Part model, mm, in its own coordinate system. A direction names the side the tool comes from. Coordinates: 2 decimals unless noted, no trailing zeros. Write each loop counter-clockwise with the first axis right and the second up, starting at its lowest first coordinate (ties: lowest second). Pieces come first, ordered by that corner, then holes. Notation, with made-up numbers: (16, -24.75) - (71, -24.75) arc R13 cw to (71, -16.75) - close; hole circle Ø1 at (-14, 43). An arc over 180 degrees is marked (long way). Write each question's results on one line, items separated by ' | '.
Autodesk Inventor part; units mm, degrees
ref_plane "YZ Plane" through (0, 0, 0) normal (1, 0, 0) x (0, 1, 0)
ref_plane "XZ Plane" through (0, 0, 0) normal (0, 1, 0) x (-1, 0, 0)
ref_plane "XY Plane" through (0, 0, 0) normal (0, 0, 1) x (1, 0, 0)
sketch "Sketch1" plane through (0, 0, 0) normal (0, 1, 0) x (-1, 0, 0)
  line L0 (-10.2591, 9.049) -> (9.7409, 9.049)
  line L1 (9.7409, 9.049) -> (9.7409, -10.951)
  line L2 (9.7409, -10.951) -> (-10.2591, -10.951)
  line L3 (-10.2591, -10.951) -> (-10.2591, 9.049)
  point P0 (0, 0)
  dimension "d0" = 20
  dimension "d1" = 20
extrude "Extrusion1" add sketch "Sketch1" along normal blind 7
sketch "Sketch2" plane through (-9.7409, 0, 9.049) normal (0, 0, 1) x (1, 0, 0)
  line L0 (20, 0) -> (0, 0)
  line L1 (20, 0) -> (20, 7)
  line L2 (0, 0) -> (0, 7)
  circle A0 centre (15, 0) radius 3.375
  circle A1 centre (5, 0) radius 3.375
  point P0 (9.7409, 0)
  dimension "d4" = 6.75
  dimension "d5" = 6.75
  dimension "d6" = 5
  dimension "d7" = 5
  dimension "d32" = 10
extrude "Extrusion2" cut sketch "Sketch2" against normal blind 7.4
sketch "Sketch3" plane through (-9.7409, 0, 1.649) normal (0, 0, 1) x (1, 0, 0)
  arc A0 (8.375, 0) -> (1.625, 0) centre (5, 0) ccw
  line L0 (18.375, 0) -> (11.625, 0)
  arc A1 (18.375, 0) -> (11.625, 0) centre (15, 0) ccw
  circle A2 centre (15, 0) radius 2.25
  circle A3 centre (5, 0) radius 2.25
  point P0 (9.7409, 0)
  dimension "d10" = 4.5
  dimension "d11" = 4.5
extrude "Extrusion3" cut sketch "Sketch3" against normal through all contours A2 L0 | L0 A2 | A3
sketch "Sketch4" plane through (0, 0, 0) normal (0, -1, 0) x (1, 0, 0)
  line L0 (-2.4909, 1.649) -> (-2.4909, -10.951)
  line L1 (3.0091, -10.951) -> (3.0091, 1.649)
  circle A0 centre (0.2591, -6.0003) radius 2.4765
  point P0 (0, 0)
  dimension "d14" = 4.953
  dimension "d15" = 5.5
  dimension "d16" = 2.75
extrude "Extrusion4" cut sketch "Sketch4" against normal through all
chamfer "Chamfer1" distance 1.905 angle 45 2 edges at (5.2591, 2.25, -10.951) (-4.7409, 2.25, -10.951)
chamfer "Chamfer2" distance 0.381 angle 45 5 edges at (-2.4909, 0, -3.6985) (-6.9909, 0, -3.6985) (7.5091, 0, -3.6985) (3.0091, 0, -3.6985) (0.2591, 7, -10.951)
chamfer "Chamfer3" distance 2.54 angle 45 4 edges at (-9.7409, 7, -0.7605) (10.2591, 7, -0.7605) (-9.7409, 3.3095, -10.951) (10.2591, 3.3095, -10.951)
sketch "Sketch5" plane through (0, 7, 0) normal (0, 1, 0) x (1, 0, 0)
  line L0 (-7.2009, 10.57) -> (7.7191, 10.57)
  circle A0 centre (0.2591, 6.0003) radius 2.4765
  line L1 (3.1554, 0.9838) -> (-2.6371, 0.9838)
  line L2 (-2.6371, 0.9838) -> (-5.5334, 6.0003)
  line L3 (-5.5334, 6.0003) -> (-2.6371, 11.0168)
  line L4 (-2.6371, 11.0168) -> (3.1554, 11.0168)
  line L5 (3.1554, 11.0168) -> (6.0517, 6.0003)
  line L6 (6.0517, 6.0003) -> (3.1554, 0.9838)
  circle A1 centre (0.2591, 6.0003) radius 5.0165
  point P0 (0, 0)
  dimension "d29" = 10.033
  dimension "d47" = 10.033
extrude "Extrusion5" cut sketch "Sketch5" against normal blind 3.175 contours A1 L0 | L0 A1
sketch "Sketch6" plane through (0, 7, 0) normal (0, 1, 0) x (1, 0, 0)
  line L0 (-7.2009, -9.049) -> (-7.2009, 10.57)
  line L1 (-7.2009, -9.049) -> (7.7191, -9.049)
  line L2 (7.7191, 10.57) -> (7.7191, -9.049)
  line L3 (-7.2009, 10.57) -> (7.7191, 10.57)
  line L4 (-4.6609, -7.144) -> (5.1791, -7.144) construction
  line L5 (-4.6609, -7.779) -> (5.1791, -7.779)
  line L6 (5.1791, -6.509) -> (-4.6609, -6.509)
  arc A0 (-4.6609, -6.509) -> (-4.6609, -7.779) centre (-4.6609, -7.144) ccw
  arc A1 (5.1791, -7.779) -> (5.1791, -6.509) centre (5.1791, -7.144) ccw
  line L7 (-4.6609, -5.239) -> (5.1791, -5.239)
  line L8 (5.1791, -3.969) -> (-4.6609, -3.969)
  arc A2 (-4.6609, -3.969) -> (-4.6609, -5.239) centre (-4.6609, -4.604) ccw
  arc A3 (5.1791, -5.239) -> (5.1791, -3.969) centre (5.1791, -4.604) ccw
  line L9 (-4.6609, -2.699) -> (5.1791, -2.699)
  line L10 (5.1791, -1.429) -> (-4.6609, -1.429)
  arc A4 (-4.6609, -1.429) -> (-4.6609, -2.699) centre (-4.6609, -2.064) ccw
  arc A5 (5.1791, -2.699) -> (5.1791, -1.429) centre (5.1791, -2.064) ccw
  point P0 (3.4133, 10.57)
  point P1 (0, 0)
  point P2 (0.2591, -7.144)
  dimension "d33" = 1.27
  dimension "d34" = 2.54
  dimension "d35" = 2.54
  dimension "d36" = 1.905
  dimension "d39" = 2.54
extrude "Extrusion6" add sketch "Sketch6" along normal blind 0.762 contours A0 L6 A1 L5 | A2 L8 A3 L7 | A4 L10 A5 L9
fillet "Fillet1" radius 0.7937 2 edges at (1.0688, 5.222, -10.951) (-0.5505, 5.222, -10.951)
move or copy body "Move Body1" bodies to move or copy 1 copy no rotation origin (0, 0, 0) rotation axis (1, 0, 0) rotation angle 90
equation "\"d16\" = 0.5 * d15"
properties part number "key_half_screw"
(1) Saw through at B-B on z = 5. Write the cut outline in (x, y).
Return value:
outline: (-9.2, -9.05) - (9.72, -9.05) - (9.72, 8.95) - (7.72, 10.95) - (4.32, 10.95) arc R0.79 ccw to (3.76, 9.59) arc R5.02 cw (long way) to (-3.25, 9.59) arc R0.79 ccw to (-3.8, 10.95) - (-7.2, 10.95) - (-9.2, 8.95) - close
(2) Saw through at C-C on y = -4.25. Write the cut outline in (x, z) (3 decimals), then the cut area to 3 significant figures.
Return value:
outline: (-9.741, 0) - (-8.116, 0) arc R3.375 cw to (-1.366, 0) - (1.884, 0) arc R3.375 cw to (8.634, 0) - (10.259, 0) - (10.259, 4.46) - (7.719, 7) - (5.706, 7) - (5.706, 7.762) - (-5.188, 7.762) - (-5.188, 7) - (-7.201, 7) - (-9.741, 4.46) - close | area: 106 mm^2
(3) Wall check: line 1 (X direction, y = 7.25, z = 1); line 2 (X direction, y = 5.75, z = 0.5); line 3 (X direction, y = -4, z = 0.5). Give the ranges that are in metal, low to high. Write a range as from..to.
Return value:
line 1: x = -9.74..-6.76, -2.73..-1.88, 2.4..3.24, 7.27..10.26 | line 2: x = -9.74..-6.93, -2.55..-2.2, 2.72..3.07, 7.45..10.26 | line 3: x = -9.74..-8.08, -1.4..1.92, 8.6..10.26
(4) Flat gauge pins, fed straight in: P1, Ø0.8, axis at x = 2.5, z = 7.5, coming from the -Y side; P2, Ø1.5, axis at y = -7, z = 6.5, coming from the -X side; P3, Ø5, axis at x = -2, y = 7.5, coming from the +Z side; P4, Ø4, axis at x = 0.26, y = 6, coming from the -Z side. Where does each tip first touch, or does it go through?
Return value:
P1: stops at y = -7.78 | P2: stops at x = -8.45 | P3: stops at z = 7 | P4: passes through
(5) Two-plate mould, pull along Y, no slides. Class faces 4 (the flat face through (8.97, 9.7, 3.36)), 5 (the flat face through (9, 0, 0)), 6 (the cylindrical face through (-0.063, 3.545, 1.886)), 7 (the flat face through (5.2, -1.649, 2.5)): released by +Y, released by -Y, zero draft, split by the parting line, or undercut.
Return value:
face 4: released by +Y | face 5: zero draft | face 6: undercut | face 7: released by -Y
(6) Saw through at A-A on y = 0. Write the cut outline in (x, z).
Return value:
outline: (-9.74, 0) - (-7.37, 0) - (-6.96, 0.38) arc R2.25 cw to (-2.52, 0.38) - (-2.11, 0) - (2.63, 0) - (3.04, 0.38) arc R2.25 cw to (7.48, 0.38) - (7.89, 0) - (10.26, 0) - (10.26, 4.46) - (7.72, 7) - (-7.2, 7) - (-9.74, 4.46) - close
(7) 3-axis set-ups, long thin cutter, end or side, ignore diameter. For faces 1 (the flat face through (0, -9.049, 4)), 2 (the cylindrical face through (5.333, -5.401, 3.374)), 3 (the cylindrical face through (-3.07, 10.47, 5.39)): which of +Z, -Z, +X, -X, +Y, -Y reach the whole face in a straight line?
Return value:
face 1: +Z, -Z, +X, -X, -Y | face 2: -Z, -Y | face 3: +Z
